```python
from build123d import *

# Parameters (mm, degrees)
EXTRUDE_1_DEPTH     = 6
SKETCH_2_R          = 2.55
CUT_EXTRUDE_1_DEPTH = 46.055521304
CUT_EXTRUDE_2_DEPTH = 46.055521304


with BuildPart() as part:
    # Эскиз1 → Бобышка-Вытянуть1 (new body)
    with BuildSketch(Plane(origin=(0, 0, 0), x_dir=(1, 0, 0), z_dir=(0, 1, 0))):
        with BuildLine():
            Line((-19, -37), (19, -37))
            ThreePointArc((19, -37), (23.242640687, -35.242640687), (25, -31))
            Line((25, -31), (25, 31))
            ThreePointArc((25, 31), (23.242640687, 35.242640687), (19, 37))
            Line((19, 37), (-19, 37))
            ThreePointArc((-19, 37), (-23.242640687, 35.242640687), (-25, 31))
            Line((-25, 31), (-25, -31))
            ThreePointArc((-25, -31), (-23.242640687, -35.242640687), (-19, -37))
        make_face()
    extrude(amount=EXTRUDE_1_DEPTH)

    # Эскиз2 → Вырез-Вытянуть1 (cut, through all)
    with BuildSketch(Plane.XZ):
        with Locations(Location((-17, -27, 0), (0, 0, 270))):
            Circle(SKETCH_2_R)
        with Locations(Location((-17, 27, 0), (0, 0, 90))):
            Circle(SKETCH_2_R)
        with BuildLine():
            Line((16, -29.55), (14, -29.55))
            ThreePointArc((14, -29.55), (11.45, -27), (14, -24.45))
            Line((14, -24.45), (16, -24.45))
            ThreePointArc((16, -24.45), (18.55, -27), (16, -29.55))
        make_face()
        with BuildLine():
            Line((16, 29.55), (14, 29.55))
            ThreePointArc((14, 29.55), (11.45, 27), (14, 24.45))
            Line((14, 24.45), (16, 24.45))
            ThreePointArc((16, 24.45), (18.55, 27), (16, 29.55))
        make_face()
    extrude(amount=-CUT_EXTRUDE_1_DEPTH, mode=Mode.SUBTRACT)

    # Эскиз3 → Вырез-Вытянуть2 (cut, through all)
    with BuildSketch(Plane.XZ):
        with BuildLine():
            Line((-25, -2), (-25, 2))
            ThreePointArc((-25, 2), (-24.414213562, 0.585786438), (-23, 0))
            ThreePointArc((-23, 0), (-24.414213562, -0.585786438), (-25, -2))
        make_face()
    extrude(amount=-CUT_EXTRUDE_2_DEPTH, mode=Mode.SUBTRACT)


solid = part.part
```
Geometry: final body of the model. Coordinates: model frame, mm. A direction names the side the tool comes from. Coordinates: 2 decimals unless noted, no trailing zeros. Order: outer loops, then holes, each group sorted by start corner. A loop starts at its lowest first (then second) coordinate and runs counter-clockwise, first axis right, second up. Notation, with made-up numbers: (30, 0) - (69, 0) arc R19 ccw to (69, 34) - close; hole circle Ø11 at (76.25, 65). An arc over 180 degrees is marked (long way). Write each question's results on one line, items separated by ' | '.
(1) Section query C-C, the plane x = 17.5. Return the cut outline in (y, z).
Values found:
outline: (0, -37) - (6, -37) - (6, -29.06) - (0, -29.06) - close; (0, -24.94) - (6, -24.94) - (6, 24.94) - (0, 24.94) - close; (0, 29.06) - (6, 29.06) - (6, 37) - (0, 37) - close
(2) Section query B-B, the plane z = 27. Return the cut outline in (x, y).
Values found:
outline: (-25, 0) - (-19.55, 0) - (-19.55, 6) - (-25, 6) - close; (-14.45, 0) - (11.45, 0) - (11.45, 6) - (-14.45, 6) - close; (18.55, 0) - (25, 0) - (25, 6) - (18.55, 6) - close
(3) Set-up query: faces 5 (the face through (15, 3, 29.55)), 6 (the face through (23.289, 2.958, -35.196)). Return all of +Z, -Z, +X, -X, +Y, -Y with unobstructed straight access to the full face (end or side cutting, diameter ignored); none if empty.
Values found:
face 5: +Y, -Y | face 6: -Z, +X, +Y, -Y
(4) First-contact query: pin 1 Ø8 at (x, z) = (-17, -27) entering from +Y. Flat tip, straight axial feed; report the tip coordinate or a pass-through.
Values found:
pin 1: stops at y = 6
(5) Line query: line 1 (X direction, y = 4.8, z = -27); line 2 (Z direction, x = 14.5, y = 5); line 3 (Z direction, x = -20, y = 5.35). Output: solid intervals per line, ascending. Write a range as [from, to].
Values found:
line 1: x = [-25, -19.55], [-14.45, 11.45], [18.55, 25] | line 2: z = [-37, -29.55], [-24.45, 24.45], [29.55, 37] | line 3: z = [-36.92, 36.92]
(6) Mould query, pull axis X, two halves, no side actions, for faces 1 (the face through (0, 0, -1)), 2 (the face through (25, 3, 0)), 3 (the face through (15, 3, 24.45)), 4 (the face through (-23.196, 2.958, -35.289)). Classes: +X half, -X half, draft (parallel to the pull), parting line (faces both ways), or undercut.
Values found:
face 1: draft | face 2: +X half | face 3: undercut | face 4: -X half
(7) Section query A-A, the plane y = 2. Return the cut outline in (x, z), plus the area to 3 significant figures.
Values found:
outline: (-25, -31) arc R6 ccw to (-19, -37) - (19, -37) arc R6 ccw to (25, -31) - (25, 31) arc R6 ccw to (19, 37) - (-19, 37) arc R6 ccw to (-25, 31) - (-25, 2) arc R2 ccw to (-23, 0) arc R2 ccw to (-25, -2) - close; hole circle Ø5.1 at (-17, -27); hole circle Ø5.1 at (-17, 27); hole (14, -29.55) - (16, -29.55) arc R2.55 ccw to (16, -24.45) - (14, -24.45) arc R2.55 ccw to start; hole (14, 24.45) - (16, 24.45) arc R2.55 ccw to (16, 29.55) - (14, 29.55) arc R2.55 ccw to start | area: 3,570 mm²
